```python
from build123d import *

# Parameters (mm, degrees)
BOSS_EXTRUDE1_DEPTH = 0.7
BOSS_EXTRUDE2_DEPTH = 28.6
SKETCH3_W           = 5
SKETCH3_H           = 1.5
BOSS_EXTRUDE3_DEPTH = 9
SKETCH4_W           = 5
SKETCH4_H           = 1.5
BOSS_EXTRUDE4_DEPTH = 9
FILLET1_R           = 1


with BuildPart() as part:
    # Sketch1 → Boss-Extrude1 (new body)
    with BuildSketch(Plane(origin=(0, 0, 0), x_dir=(1, 0, 0), z_dir=(0, 1, 0))):
        with BuildLine():
            Line((-17.5, 0), (-17.5, 18.884045511))
            ThreePointArc((-17.5, 18.884045511), (-16.837918728, 21.370501041), (-15.027015558, 23.198462316))
            Line((-15.027015558, 23.198462316), (-1.516209335, 31.111934533))
            ThreePointArc((-1.516209335, 31.111934533), (0, 31.523284449), (1.516209335, 31.111934533))
            Line((1.516209335, 31.111934533), (15.027015558, 23.198462316))
            ThreePointArc((15.027015558, 23.198462316), (16.837918728, 21.370501041), (17.5, 18.884045511))
            Line((17.5, 18.884045511), (17.5, 0))
            Line((17.5, 0), (17.5, -18.884045511))
            ThreePointArc((17.5, -18.884045511), (16.837918728, -21.370501041), (15.027015558, -23.198462316))
            Line((15.027015558, -23.198462316), (1.516209335, -31.111934533))
            ThreePointArc((1.516209335, -31.111934533), (0, -31.523284449), (-1.516209335, -31.111934533))
            Line((-1.516209335, -31.111934533), (-15.027015558, -23.198462316))
            ThreePointArc((-15.027015558, -23.198462316), (-16.837918728, -21.370501041), (-17.5, -18.884045511))
            Line((-17.5, -18.884045511), (-17.5, 0))
        make_face()
        with BuildLine():
            Line((2.65, 27.5), (2.65, 26.5))
            ThreePointArc((2.65, 26.5), (0, 23.85), (-2.65, 26.5))
            Line((-2.65, 26.5), (-2.65, 27.5))
            ThreePointArc((-2.65, 27.5), (0, 30.15), (2.65, 27.5))
        make_face(mode=Mode.SUBTRACT)
        with BuildLine():
            Line((2.65, -26.5), (2.65, -27.5))
            ThreePointArc((2.65, -27.5), (0, -30.15), (-2.65, -27.5))
            Line((-2.65, -27.5), (-2.65, -26.5))
            ThreePointArc((-2.65, -26.5), (0, -23.85), (2.65, -26.5))
        make_face(mode=Mode.SUBTRACT)
    extrude(amount=BOSS_EXTRUDE1_DEPTH)

    # Sketch2 → Boss-Extrude2 (add)
    with BuildSketch(Plane(origin=(0, 0.7, 0), x_dir=(1, 0, 0), z_dir=(0, 1, 0))):
        with BuildLine():
            Line((-12.25, 21.75), (12.25, 21.75))
            ThreePointArc((12.25, 21.75), (15.078427125, 20.578427125), (16.25, 17.75))
            Line((16.25, 17.75), (16.25, -17.75))
            ThreePointArc((16.25, -17.75), (15.078427125, -20.578427125), (12.25, -21.75))
            Line((12.25, -21.75), (-12.25, -21.75))
            ThreePointArc((-12.25, -21.75), (-15.078427125, -20.578427125), (-16.25, -17.75))
            Line((-16.25, -17.75), (-16.25, 17.75))
            ThreePointArc((-16.25, 17.75), (-15.078427125, 20.578427125), (-12.25, 21.75))
        make_face()
    extrude(amount=BOSS_EXTRUDE2_DEPTH)

    # Sketch3 → Boss-Extrude3 (add)
    with BuildSketch(Plane.ZY.offset(16.25)):
        with Locations((-10.5, 10)):
            Rectangle(SKETCH3_W, SKETCH3_H)
        with Locations((10.5, 10)):
            Rectangle(SKETCH3_W, SKETCH3_H)
        with Locations((0, 19.18013067)):
            Rectangle(SKETCH3_W, SKETCH3_H)
    extrude(amount=BOSS_EXTRUDE3_DEPTH)

    # Sketch4 → Boss-Extrude4 (add)
    with BuildSketch(Plane(origin=(16.25, 0, 0), x_dir=(0, 0, -1), z_dir=(1, 0, 0))):
        with Locations((-9, 15.7)):
            Rectangle(SKETCH4_W, SKETCH4_H)
        with Locations((9, 15.7)):
            Rectangle(SKETCH4_W, SKETCH4_H)
    extrude(amount=BOSS_EXTRUDE4_DEPTH)

    # Fillet1
    fillet1_edges = [part.edges().sort_by_distance(p)[0] for p in [
        (-15.078427125, 29.3, 20.578427125),
        (0, 29.3, 21.75),
        (15.078427125, 29.3, 20.578427125),
        (16.25, 29.3, 0),
        (15.078427125, 29.3, -20.578427125),
        (0, 29.3, -21.75),
        (-15.078427125, 29.3, -20.578427125),
        (-16.25, 29.3, 0),
    ]]
    fillet(fillet1_edges, radius=FILLET1_R)


solid = part.part
```
The listing builds one solid part. Answer for the finished solid, in the listing's coordinates (mm). A direction names the side the tool comes from. Coordinates: 2 decimals unless noted, no trailing zeros. Order: outer loops, then holes, each group sorted by start corner. A loop starts at its lowest first (then second) coordinate and runs counter-clockwise, first axis right, second up. Notation, with made-up numbers: M -11.75,39 L 44.25,39 A24 cw 44.25,72 Z; hole C 52.25,59.5 d1. An arc over 180 degrees is marked long. Answer as a JSON object with one key per item and string values. Group by question number.
1. Flat-ended cylindrical pins translate along their axes: P1, Ø0.6, axis at y = 0.5, z = -1.5, coming from the +X side; P2, Ø1.5, axis at x = -23, z = 1, coming from the +Y side; P3, Ø5, axis at x = -9, y = 12, coming from the -Z side. Find the tip coordinate at first contact, or state that the pin passes through.
2. Section B-B on z = 16 is taken. Write down the section's boundary in (x, y), then the cut area to 3 significant figures.
3. Straight lines are drawn through the part: line 1 (Z direction, x = 5, y = 18.5); line 2 (Y direction, x = -22, z = 10); line 3 (X direction, y = 5.75, z = 9.5). For each, find the intervals that lie inside material, in ascending order.
4. Section A-A on x = 0 is taken. Write down the section's boundary in (y, z), then the cut area to 3 significant figures.
5. A tool of negligible diameter and unlimited length cuts with its end or side. For faces 1 (the flat face through (-21, 10.75, -11)), 2 (the flat face through (0, 14, -21.75)), 3 (the flat face through (21, 16.45, 9)), from which of +Z, -Z, +X, -X, +Y, -Y can it reach the whole face along a straight path? Write none if from no direction.
6. Section C-C on y = 4.25 is taken. Write down the section's boundary in (x, z), then the cut area to 3 significant figures.
7. Determine the mould class of faces 4 (the flat face through (21, 16, -11.5)), 5 (the cylindrical face through (0.06, 0.35, 30.15)), 6 (the cylindrical face through (-0.06, 0.35, 23.85)), 7 (the flat face through (25.25, 16, -9)) for opening direction X: released by +X, released by -X, zero draft, split by the parting line, or undercut.
8. Section D-D on z = 25 is taken. Write down the section's boundary in (x, y), then the cut area to 3 significant figures.
Values follow:
{
 "1": {"P1": "x = 17.5", "P2": "y = 19.93", "P3": "z = -21.75"},
 "2": {"outline": "M -17.5,0 L 17.5,0 L 17.5,0.7 L 16.25,0.7 L 16.25,28.3 A1 ccw 15.25,29.3 L -15.25,29.3 A1 ccw -16.25,28.3 L -16.25,0.7 L -17.5,0.7 Z", "area": "954 mm2"},
 "3": {"line 1": "-21.75 to 21.75", "line 2": "9.25 to 10.75", "line 3": "-16.25 to 16.25"},
 "4": {"outline": "M 0,-31.52 L 0.7,-31.52 L 0.7,-30.15 L 0,-30.15 Z; M 0,-23.85 L 0.7,-23.85 L 0.7,-21.75 L 28.3,-21.75 A1 ccw 29.3,-20.75 L 29.3,20.75 A1 ccw 28.3,21.75 L 0.7,21.75 L 0.7,23.85 L 0,23.85 Z; M 0,30.15 L 0.7,30.15 L 0.7,31.52 L 0,31.52 Z", "area": "1,280 mm2"},
 "5": {"face 1": "+Z, -Z, -X, +Y", "face 2": "-Z, +X, -X, +Y", "face 3": "+Z, -Z, +X, +Y"},
 "6": {"outline": "M -16.25,-17.75 A4 ccw -12.25,-21.75 L 12.25,-21.75 A4 ccw 16.25,-17.75 L 16.25,17.75 A4 ccw 12.25,21.75 L -12.25,21.75 A4 ccw -16.25,17.75 Z", "area": "1,400 mm2"},
 "7": {"face 4": "zero draft", "face 5": "undercut", "face 6": "undercut", "face 7": "released by +X"},
 "8": {"outline": "M -11.95,0 L -2.18,0 L -2.18,0.7 L -11.95,0.7 Z; M 2.18,0 L 11.95,0 L 11.95,0.7 L 2.18,0.7 Z", "area": "13.7 mm2"}
}
